Autodesk Inventor part; units mm, degrees
ref_plane "XY Plane" through (0, 0, 0) normal (0, 0, 1) x (1, 0, 0)
sketch "Skizze1" plane through (0, 0, 0) normal (0, 0, 1) x (1, 0, 0)
  line L0 (-75, 75) -> (75, 75)
  line L1 (75, 75) -> (75, -75)
  line L2 (75, -75) -> (-75, -75)
  line L3 (-75, -75) -> (-75, 75)
  line L4 (-75, 75) -> (75, -75) construction
  line L5 (75, 75) -> (-75, -75) construction
  point P0 (0, 0)
  dimension "d0" = 150
  dimension "d1" = 150
extrude "Extrusion1" add sketch "Skizze1" along normal mid plane 20
sketch "Skizze5" plane through (0, 0, -10) normal (0, 0, -1) x (-1, 0, 0)
  line L0 (-75, -75) -> (75, -75)
  line L1 (75, -75) -> (75, 75)
  line L2 (75, 75) -> (-75, 75)
  line L3 (-75, 75) -> (-75, -75)
  circle A0 centre (0, 0) radius 13
  dimension "d30" = 26
extrude "Extrusion3" cut sketch "Skizze5" against normal blind 6 contours A0
chamfer "Fasen2" distance 2 angle 45 4 edges at (-75, -75, 0) (75, -75, 0) (-75, 75, 0) (75, 75, 0)
chamfer "Fasen3" distance 0.5 angle 45 1 edges at (13, 0, -10)
sketch "Skizze6" plane through (0, 0, -4) normal (0, 0, -1) x (-1, 0, 0)
  circle A0 centre (0, 0) radius 13
hole "Bohrung3" at (0, 0, -4) direction (0, 0, 1) diameter 4.134 end through all
sketch "Skizze7" plane through (0, 0, -10) normal (0, 0, -1) x (-1, 0, 0)
  line L0 (-75, 73) -> (-73, 75)
  line L1 (-75, 73) -> (-75, -73)
  line L2 (-73, -75) -> (-75, -73)
  line L3 (-73, -75) -> (73, -75)
  line L4 (75, -73) -> (73, -75)
  line L5 (75, -73) -> (75, 73)
  line L6 (73, 75) -> (75, 73)
  line L7 (73, 75) -> (-73, 75)
  circle A0 centre (0, 0) radius 13.5
  point P0 (0, -24)
  dimension "d46" = 24
  dimension "d47" = 0
hole "Bohrung4" at (0, -24, -10) direction (0, 0, 1) diameter 5.5 end through all counterbore diameter 10 counterbore depth 5
pattern_circular "Runde Anordnung2" count 4 over 360 about axis through (0, 0, -10) along (0, 0, 1) of "Bohrung4"
chamfer "Fasen4" distance 0.5 angle 45 4 edges at (0, -29, -10) (29, 0, -10) (0, 29, -10) (-29, 0, -10)
chamfer "Fasen5" distance 0.5 angle 45 4 edges at (26.75, 0, 10) (0, 26.75, 10) (-26.75, 0, 10) (0, -26.75, 10)
chamfer "Fasen6" distance 0.5 angle 45 1 edges at (0, -2.067, 10)
chamfer "Fasen7" distance 0.5 angle 45 1 edges at (0, -2.067, -4)
properties part number "Koordinaten-Platte"
Can you work these out from the model? Positions are in its coordinate system, mm. A direction names the side the tool comes from. Give positions to 0.01 mm unless a question says otherwise; leave off trailing zeros. Order: outer loops, then holes, each group sorted by start corner. A loop starts at its lowest first (then second) coordinate and runs counter-clockwise, first axis right, second up. Notation, with made-up numbers: M 0.25,46.5 L 34.25,46.5 A5 cw 34.25,52.5 Z; hole C 62,57 d11. An arc over 180 degrees is marked long. Use a Markdown table: item, result. Add a question column.
Item 1: If I drill on L1, parallel to X at y = -24, z = -5.85; L2, parallel to X at y = -24, z = 4.5, over which ranges is the centre line in solid material (lowest first)? Write a range as [from, to].
Item 2: Suppose I cut it at C-C (x = 0). Count the separate pieces of the cut face and the enclosed holes in it, then the cut area to 3 significant figures.
Item 3: Suppose I cut it at A-A (y = -24). List the corners of the cut face in (x, z) for me.
Item 4: Will these pins go through, and if not, where does the flat tip stop? pin 1 (8 mm diameter, centred on x = -24.5, y = -1, fed in from -Z); pin 2 (3.5 mm diameter, centred on x = 0, y = 0, fed in from -Z); pin 3 (5 mm diameter, centred on x = -1, y = 23, fed in from -Z); pin 4 (6 mm diameter, centred on x = -24, y = 0, fed in from +Z).
Item 5: For faces 1 (the cylindrical face through (-0.121, -26.747, 2.351)), 2 (the cylindrical face through (0, -29, -7)), which set-ups out of +Z, -Z, +X, -X, +Y, -Y let a thin tool reach every point of the face, with its end or its side?
Item 6: We'd pull the mould along Y, two halves only. Please class faces 3 (the flat face through (-1, 18, 10)), 4 (the cylindrical face through (10.316, -7.91, -6.788)), 5 (the flat face through (1, -75, 0)): +Y half, -Y half, draft (parallel to the pull), parting line (faces both ways), or undercut.
Answer sheet:
| question | item | result |
|---|---|---|
| 1 | L1 | x = [-75, -5], [5, 75] |
| 1 | L2 | x = [-75, -2.75], [2.75, 75] |
| 2 | separate pieces | 4 |
| 2 | enclosed holes | 0 |
| 2 | area | 2,520 mm² |
| 3 | outline | M -75,-10 L -5.5,-10 L -5,-9.5 L -5,-5 L -2.75,-5 L -2.75,9.5 L -3.25,10 L -75,10 Z; M 2.75,-5 L 5,-5 L 5,-9.5 L 5.5,-10 L 75,-10 L 75,10 L 3.25,10 L 2.75,9.5 Z |
| 4 | pin 1 | stops at z = -9.62 |
| 4 | pin 2 | passes through |
| 4 | pin 3 | stops at z = -5 |
| 4 | pin 4 | stops at z = 9.75 |
| 5 | face 1 | +Z, -Z |
| 5 | face 2 | -Z |
| 6 | face 3 | draft |
| 6 | face 4 | undercut |
| 6 | face 5 | -Y half |
